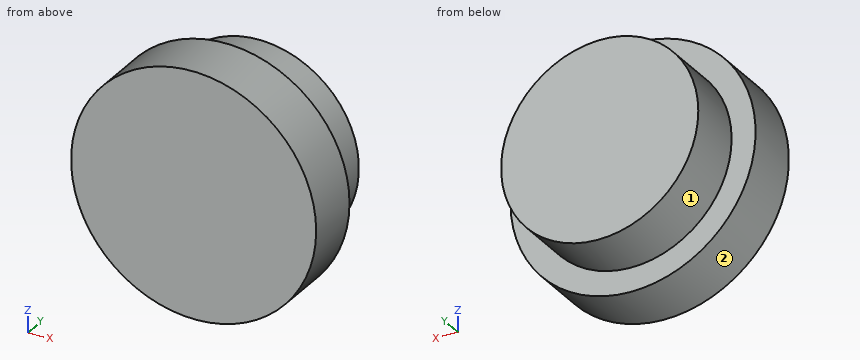
from build123d import *

# Parameters (mm, degrees)
F0_R     = 55.201714
F1_DEPTH = 25.4
F2_R     = 44.416682
F4_DEPTH = 25.4
F3_R     = 44.416682
F5_DEPTH = 25.4
F6_R     = 35.177102
F8_DEPTH = 50.8


with BuildPart() as f1:
    # F0 (on Front) → F1 (new body)
    with BuildSketch(Plane.XZ):
        Circle(F0_R)
    extrude(amount=F1_DEPTH)

    # F2 (on Front) → F4 (join)
    with BuildSketch(Plane.XZ):
        Circle(F2_R)
    extrude(amount=F4_DEPTH)

    # F3 (on face) → F5 (join)
    with BuildSketch(Plane(origin=(0, 25.4, 0), x_dir=(-1, 0, 0), z_dir=(0, 1, 0))):
        Circle(F3_R)
    extrude(amount=-F5_DEPTH)

    # F6 (on face) → F8 (join)
    with BuildSketch(Plane(origin=(0, 25.4, 0), x_dir=(-1, 0, 0), z_dir=(0, 1, 0))):
        Circle(F6_R)
    extrude(amount=-F8_DEPTH)


solid = f1.part
Geometry check sheet. Reference: the model listing, model coordinates, mm. Face numbers are marked on the shaded views. A direction names the side the tool comes from. Round coordinates to 2 decimals unless told otherwise and drop trailing zeros. Order: outer loops, then holes, each group sorted by start corner. A loop starts at its lowest first (then second) coordinate and runs counter-clockwise, first axis right, second up. Notation, with made-up numbers: (31, -31.5) -> (60, -31.5) arc R30 cw to (60, 7.5) -> close; hole circle Ø5 at (-6, 6.25). An arc over 180 degrees is marked (long way). Use one line per item in the form item = value.
1. Cross-section at B-B, the plane x = 0. Enter the section's corners in (y, z).
Working result:
outline = (-25.4, -55.2) -> (0, -55.2) -> (0, -44.42) -> (25.4, -44.42) -> (25.4, 44.42) -> (0, 44.42) -> (0, 55.2) -> (-25.4, 55.2) -> close
2. Cross-section at D-D, the plane y = -19. Enter the section's corners in (x, z), plus the area to 3 significant figures.
Working result:
outline = circle Ø110.4 at (0, 0)
area = 9,570 mm^2
3. Cross-section at C-C, the plane y = 18. Enter the section's corners in (x, z).
Working result:
outline = circle Ø88.83 at (0, 0)
4. Set-up check for the marked faces 1 and 2: record each of +Z, -Z, +X, -X, +Y, -Y from which the full face is reachable in a straight line by a thin tool's end or side.
Working result:
face_1 = +Y
face_2 = +Y, -Y
5. Cross-section at A-A, the plane z = 0. Enter the section's corners in (x, y).
Working result:
outline = (-55.2, -25.4) -> (55.2, -25.4) -> (55.2, 0) -> (44.42, 0) -> (44.42, 25.4) -> (-44.42, 25.4) -> (-44.42, 0) -> (-55.2, 0) -> close
6. Scan lines: line 1 along Y through (x, z) = (47.5, -7); line 2 along X through (y, z) = (7, -0.5); line 3 along Z through (x, y) = (15, -22). Record each from-to range of solid material in increasing order. Write a range as from..to.
Working result:
line_1 = -25.4..0
line_2 = -44.41..44.41
line_3 = -53.12..53.12
7. Go/stop test with flat-tipped pins: pin 1 (5 mm diameter, centred on x = 42.5, y = -6, fed in from -Z); pin 2 (6 mm diameter, centred on x = 0.5, y = 0, fed in from +Z); pin 3 (8 mm diameter, centred on y = -14.5, z = -12, fed in from +X). Record where each tip stops, or that it passes through.
Working result:
pin_1 = -38.04
pin_2 = 55.2
pin_3 = 54.62
